from build123d import *

# Parameters (mm, degrees)
THREAD_ENVELOPE_START = -7
PROFILE_1_R           = 1.5
THREAD_ENVELOPE_DEPTH = 7
PROFILE_2_R           = 2.75
SOCKET_HEAD_DEPTH     = 3


with BuildPart() as part:
    # Profile_1 → Thread_envelope (new body)
    with BuildSketch(Plane.XY.offset(THREAD_ENVELOPE_START)):
        Circle(PROFILE_1_R)
    extrude(amount=THREAD_ENVELOPE_DEPTH)

    # Profile_2 → Socket_head (add)
    with BuildSketch(Plane.XY):
        Circle(PROFILE_2_R)
        Polygon((1.25, 0.721687836), (0, 1.443375673), (-1.25, 0.721687836), (-1.25, -0.721687836), (0, -1.443375673), (1.25, -0.721687836), align=None, mode=Mode.SUBTRACT)
    extrude(amount=SOCKET_HEAD_DEPTH)


solid = part.part
Design review of the part built by this model. Coordinates are the model's own, in mm. A direction names the side the tool comes from. Round coordinates to 2 decimals unless told otherwise and drop trailing zeros. Order: outer loops, then holes, each group sorted by start corner. A loop starts at its lowest first (then second) coordinate and runs counter-clockwise, first axis right, second up. Notation, with made-up numbers: M 29,16 L 37,16 A27 ccw 37,38 Z; hole C 69,2.25 d9. An arc over 180 degrees is marked long. Answer as CSV lines item,"result". Start each with the question number.
1) For pin 1 Ø1 at (x, z) = (-1.5, 2) entering from -Y; pin 2 Ø3 at (y, z) = (1, -4) entering from -X, all flat-tipped, find the tip position at first contact; note any pin that passes through.
2) Add section D-D (x = 1.8). Give the boundary of the cut face in (y, z), then the cut area to 3 significant figures.
3) Wall thickness on line 1 along X through (y, z) = (0.05, 2.25); line 2 along Z through (x, y) = (-1.1, 2); line 3 along Z through (x, y) = (0.7, 0.6): over which ranges is each line inside the solid? List them lowest first. Write a range as [from, to].
4) Add section B-B (y = 0). Give the boundary of the cut face in (x, z).
5) The part is to be moulded in two halves that separate along Y. For faces 1 (the face through (-1.25, 0, 1)), 2 (the face through (0, 0, -7)), 3 (the face through (-1.5, 0.07, -3.55)), 4 (the face through (0.616, -1.088, 1.479)), say which applies: +Y half, -Y half, draft (parallel to the pull), parting line (faces both ways), or undercut.
6) Add section C-C (z = -1). Give the boundary of the cut face in (x, y), then the cut area to 3 significant figures.
7) Add section A-A (z = 2). Give the boundary of the cut face in (x, y), then the cut area to 3 significant figures.
8) Tool access review of faces 5 (the face through (1.2, -1.2, 0)), 6 (the face through (-0.616, 1.088, 1.479)), 7 (the face through (-0.596, -2.685, 1.479)): name each direction out of +Z, -Z, +X, -X, +Y, -Y from which nothing blocks a thin tool from reaching the whole face with its end or side.
Resolved:
1,pin 1,"y = -2.56"
1,pin 2,"x = -1.5"
2,outline,"M -2.08,0 L 2.08,0 L 2.08,3 L -2.08,3 Z"
2,area,"12.5 mm^2"
3,line 1,"[-2.75, -1.25], [1.25, 2.75]"
3,line 2,"[0, 3]"
3,line 3,"[-7, 0]"
4,outline,"M -2.75,0 L -1.5,0 L -1.5,-7 L 1.5,-7 L 1.5,0 L 2.75,0 L 2.75,3 L 1.25,3 L 1.25,0 L -1.25,0 L -1.25,3 L -2.75,3 Z"
5,face 1,"undercut"
5,face 2,"draft"
5,face 3,"parting line"
5,face 4,"undercut"
6,outline,"C 0,0 d3"
6,area,"7.07 mm^2"
7,outline,"C 0,0 d5.5; hole M -1.25,-0.72 L 0,-1.44 L 1.25,-0.72 L 1.25,0.72 L 0,1.44 L -1.25,0.72 Z"
7,area,"18.3 mm^2"
8,face 5,"-Z"
8,face 6,"+Z"
8,face 7,"+Z, -Z"
